Source: CAD feature listing. Evaluate the final solid. Frame: model axes, mm. A direction names the side the tool comes from. Coordinates: 2 decimals unless noted, no trailing zeros. Loops run counter-clockwise (first coordinate to the right, second up) from the corner with the lowest first, then second, coordinate; pieces in that order, holes last. Notation, with made-up numbers: (-27.75, 7.5) -> (-3.75, 7.5) arc R17 ccw to (-3.75, 22.5) -> close; hole circle Ø3 at (-12.5, 70). An arc over 180 degrees is marked (long way). Answer as CSV lines item,"result".
Autodesk Inventor part; units mm, degrees
ref_plane "YZ Plane" through (0, 0, 0) normal (1, 0, 0) x (0, 1, 0)
ref_plane "XZ Plane" through (0, 0, 0) normal (0, 1, 0) x (-1, 0, 0)
ref_plane "XY Plane" through (0, 0, 0) normal (0, 0, 1) x (1, 0, 0)
sketch "Sketch1" plane through (0, 0, 0) normal (0, 1, 0) x (-1, 0, 0)
  line L0 (0, 57.15) -> (-25.5, 57.15)
  line L1 (-25.5, 57.15) -> (-76.5, 44.45)
  line L2 (-76.5, 44.45) -> (-102, 44.45)
  line L3 (-102, 0) -> (0, 0)
  line L4 (-102, 42.45) -> (-76.2547, 42.45)
  line L5 (-76.2547, 42.45) -> (-25.2547, 55.15)
  line L6 (-25.2547, 55.15) -> (0, 55.15)
  line L7 (-102, 0) -> (-102, 42.45) construction
  line L8 (-102, 44.45) -> (-102, 42.45)
  line L9 (0, 57.15) -> (0, 55.15)
  line L10 (0, 0) -> (0, 55.15) construction
  dimension "d0" = 114.3
  dimension "d1" = 88.9
  dimension "d2" = 2
  dimension "d3" = 2
  dimension "d4" = 102
  dimension "d5" = 25.5
  dimension "d6" = 25.5
  dimension "d7" = 2
revolve "Revolution1" add sketch "Sketch1" angle 360 about axis through (102, 0, 0) along (-1, 0, 0)
equation "\"d0\" = D"
equation "\"d1\" = D1"
equation "\"d2\" = T"
equation "\"d3\" = T1"
equation "\"d4\" = L"
equation "\"d5\" = 0.25 * L"
equation "\"d6\" = 0.25 * L"
equation "\"d7\" = T"
equation "\"T\" = 2"
equation "\"D\" = 114.3"
equation "\"D1\" = 88.9"
equation "\"L\" = 102"
equation "\"T1\" = 2"
equation "\"Size_Designation\" = 1.2345"
properties part number "ISO 5251 Concentric reducers DN100 x DN80 2" material "Stainless Steel"
(1) Cut plane D-D (x = 63). Return the cut outline in (y, z).
Computed values:
outline,"circle Ø95.62 at (0, 0); hole circle Ø91.5 at (0, 0)"
(2) Draft query along Y for faces 1 (the conical face through (61.976, 14.438, 45.847)), 2 (the conical face through (61.73, -44.97, -9.99)), 3 (the flat face through (102, -36, 23)). Return one class per face: released by +Y, released by -Y, zero draft, split by the parting line, or undercut.
Computed values:
face 1,"split by the parting line"
face 2,"undercut"
face 3,"zero draft"
(3) Pin query (flat end, axial travel): pin 1 Ø12 at (x, z) = (15.5, -12.5) entering from +Y; pin 2 Ø6 at (x, z) = (25.5, 8) entering from +Y; pin 3 Ø3 at (x, z) = (33, -9) entering from -Y. Return the tip coordinate at first contact, or that it passes through.
Computed values:
pin 1,"y = 56.78"
pin 2,"y = 56.93"
pin 3,"y = -54.99"
(4) Material intervals for L1, parallel to Y at x = 10.25, z = 0; L2, parallel to Z at x = 94.5, y = 1; L3, parallel to Y at x = 37, z = 36.5, sorted ascending. Write a range as [from, to].
Computed values:
L1,"[-57.15, -55.15], [55.15, 57.15]"
L2,"[-44.44, -42.44], [42.44, 44.44]"
L3,"[-40.18, -37.35], [37.35, 40.18]"
(5) Cut plane A-A (y = 0). Return the cut outline in (x, z), then the cut area to 3 significant figures.
Computed values:
outline,"(0, -57.15) -> (25.5, -57.15) -> (76.5, -44.45) -> (102, -44.45) -> (102, -42.45) -> (76.25, -42.45) -> (25.25, -55.15) -> (0, -55.15) -> close; (0, 55.15) -> (25.25, 55.15) -> (76.25, 42.45) -> (102, 42.45) -> (102, 44.45) -> (76.5, 44.45) -> (25.5, 57.15) -> (0, 57.15) -> close"
area,"414 mm^2"
(6) Access query for faces 4 (the flat face through (0, 30, -47)), 5 (the cylindrical face through (12.451, -33.558, -43.765)), 6 (the cylindrical face through (89.428, -13.352, 42.397)). Directions: +Z, -Z, +X, -X, +Y, -Y. A direction counts if a zero-diameter tool reaches every point of the face in a straight line with its end or side. Return the directions, or none.
Computed values:
face 4,"+Z, -Z, -X, +Y, -Y"
face 5,"-X"
face 6,"+X"
(7) Cut plane C-C (x = 16.5). Return the cut outline in (y, z).
Computed values:
outline,"circle Ø114.3 at (0, 0); hole circle Ø110.3 at (0, 0)"
